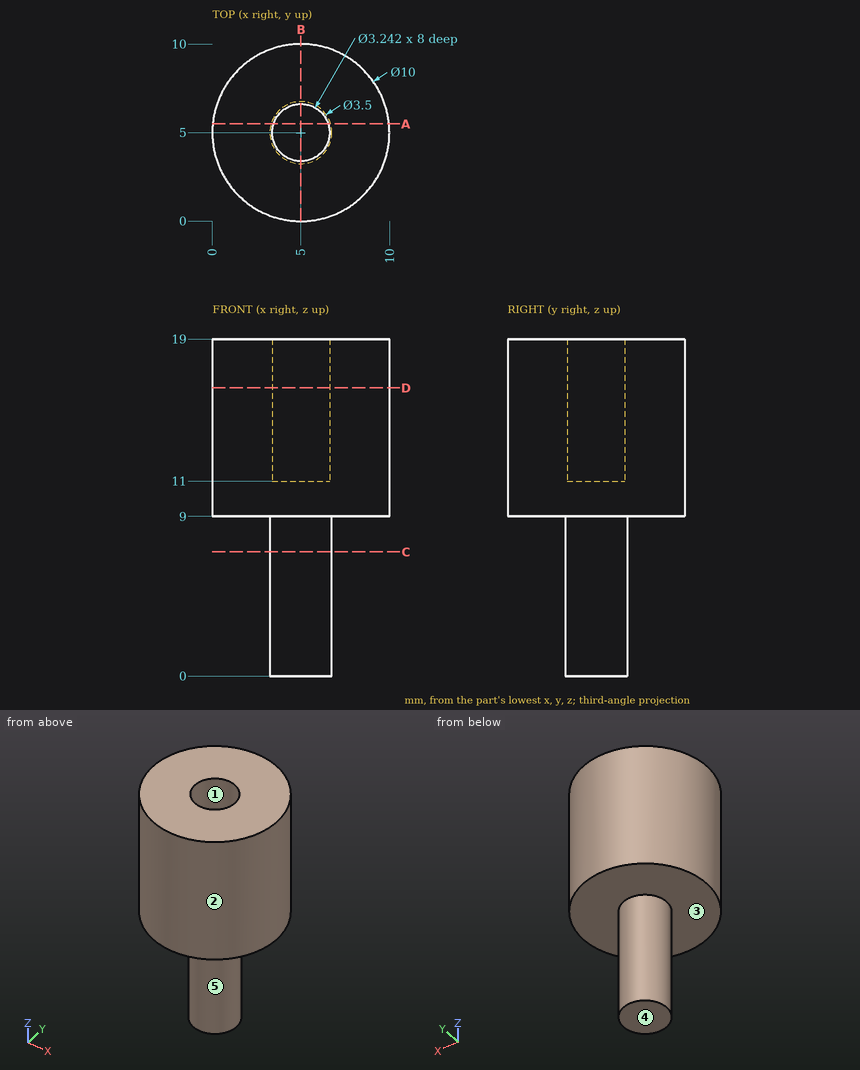
Print and shaded views of the part. All mm, measured from the part's lowest x, y and z. A direction names the side the tool comes from. Coordinates: 2 decimals unless noted, no trailing zeros. Order: outer loops, then holes, each group sorted by start corner. A loop starts at its lowest first (then second) coordinate and runs counter-clockwise, first axis right, second up. Notation, with made-up numbers: (-14, 57.25) -> (37, 57.25) arc R23 cw to (37, 68.25) -> close; hole circle Ø2 at (7.5, 7.25). An arc over 180 degrees is marked (long way). Use one line per item in the form item = value. Start each with the question number.
1) Drill centre lines: L1, parallel to Y at x = 5, z = 17; L2, parallel to Z at x = 1.5, y = 4.75; L3, parallel to Z at x = 6, y = 5.5. Where is each one in solid material? Low to high. Write a range as [from, to].
2) Band-saw the part on D-D on z = 16.25. Give the cut face in (x, y).
3) Band-saw the part on C-C on z = 7. Give the cut face in (x, y).
4) Band-saw the part on A-A on y = 5.5. Give the cut face in (x, z).
5) Drop flat-ended pins along their axis: pin 1 (1.5 mm diameter, centred on x = 8.5, z = 11, fed in from -Y); pin 2 (5 mm diameter, centred on x = 2.5, z = 13.5, fed in from +Y); pin 3 (1.6 mm diameter, centred on x = 4.5, y = 4.5, fed in from +Z); pin 4 (5 mm diameter, centred on y = 3, z = 4.5, fed in from -X). Give the stop position or say it passes through.
6) Pull direction Y, two halves, no side cores. Call the marked faces 1, 2 and 3: +Y half, -Y half, draft (parallel to the pull), parting line (faces both ways), or undercut.
7) Tool access for the marked faces 4 and 5: list every direction of +Z, -Z, +X, -X, +Y, -Y with a clear straight run to the whole face (end or side of a thin tool).
8) Band-saw the part on B-B on x = 5. Give the cut face in (y, z), then the cut area to 3 significant figures.
Entries:
q1.L1 = [0, 3.38], [6.62, 10]
q1.L2 = [9, 19]
q1.L3 = [0, 11]
q2.outline = circle Ø10 at (5, 5); hole circle Ø3.24 at (5, 5)
q3.outline = circle Ø3.5 at (5, 5)
q4.outline = (0.03, 9) -> (3.32, 9) -> (3.32, 0) -> (6.68, 0) -> (6.68, 9) -> (9.97, 9) -> (9.97, 19) -> (6.54, 19) -> (6.54, 11) -> (3.46, 11) -> (3.46, 19) -> (0.03, 19) -> close
q5.pin_1 = 0.82
q5.pin_2 = 10
q5.pin_3 = 11
q5.pin_4 = 3.25
q6.face_1 = undercut
q6.face_2 = parting line
q6.face_3 = draft
q7.face_4 = -Z, +X, -X, +Y, -Y
q7.face_5 = -Z
q8.outline = (0, 9) -> (3.25, 9) -> (3.25, 0) -> (6.75, 0) -> (6.75, 9) -> (10, 9) -> (10, 19) -> (6.62, 19) -> (6.62, 11) -> (3.38, 11) -> (3.38, 19) -> (0, 19) -> close
q8.area = 106 mm2
